Geometry check sheet. Reference: the model listing, model coordinates, mm. Face numbers are marked on the shaded views. A direction names the side the tool comes from. Coordinates: 2 decimals unless noted, no trailing zeros. Loops run counter-clockwise (first coordinate to the right, second up) from the corner with the lowest first, then second, coordinate; pieces in that order, holes last. Notation, with made-up numbers: (-30.5, 60.5) - (-2.5, 60.5) arc R19 cw to (-2.5, 92.5) - close; hole circle Ø11 at (70, 77.25). An arc over 180 degrees is marked (long way). One line per item, written item: value.
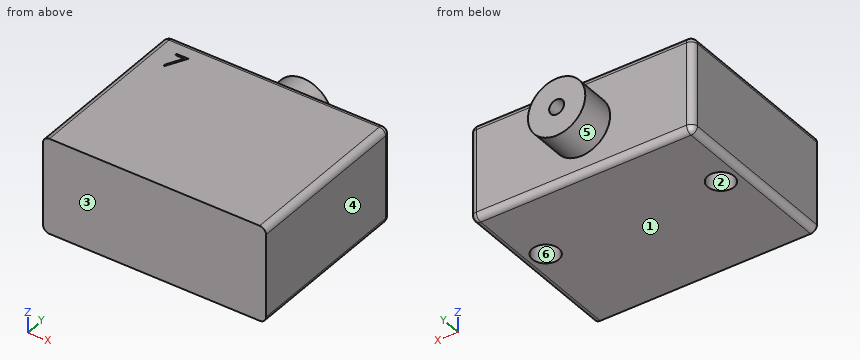
from build123d import *

# Parameters (mm, degrees)
CROQUIS1_W              = 70
CROQUIS1_H              = 30
SALIENTE_EXTRUIR1_DEPTH = 55
CROQUIS9_R              = 4.15
CORTAR_EXTRUIR6_DEPTH   = 27
REDONDEO1_R             = 2
CORTAR_EXTRUIR9_DEPTH   = 1
CROQUIS13_R             = 9
SALIENTE_EXTRUIR2_DEPTH = 11
CROQUIS14_R             = 2.35
CORTAR_EXTRUIR10_DEPTH  = 44


with BuildPart() as part:
    # Croquis1 → Saliente-Extruir1 (new body)
    with BuildSketch(Plane(origin=(0, 0, 0), x_dir=(1, 0, 0), z_dir=(0, 1, 0))):
        Rectangle(CROQUIS1_W, CROQUIS1_H)
    extrude(amount=SALIENTE_EXTRUIR1_DEPTH)

    # Croquis9 → Cortar-Extruir6 (cut)
    with BuildSketch(Plane(origin=(0, 0, -15), x_dir=(-1, 0, 0), z_dir=(0, 0, -1))):
        with Locations((-27.5, 32)):
            Circle(CROQUIS9_R)
        with Locations((27.5, 32)):
            Circle(CROQUIS9_R)
    extrude(amount=-CORTAR_EXTRUIR6_DEPTH, mode=Mode.SUBTRACT)

    # Redondeo1
    redondeo1_edges = [part.edges().sort_by_distance(p)[0] for p in [
        (-35, 55, 0),
        (0, 55, 15),
        (35, 55, 0),
        (0, 55, -15),
        (35, 27.5, 15),
        (-35, 27.5, 15),
        (-35, 27.5, -15),
        (35, 27.5, -15),
    ]]
    fillet(redondeo1_edges, radius=REDONDEO1_R)

    # Croquis12 → Cortar-Extruir9 (cut)
    with BuildSketch(Plane.XY.offset(15)):
        Polygon((-27.897004406, 49.221392525), (-24.204696713, 49.221392525), (-27.358542867, 43.067546371), (-27.823687098, 43.323555986), (-25.115754406, 48.606007909), (-27.897004406, 48.606007909), align=None)
    extrude(amount=-CORTAR_EXTRUIR9_DEPTH, mode=Mode.SUBTRACT)

    # Croquis13 → Saliente-Extruir2 (add)
    with BuildSketch(Plane(origin=(0, 55, 0), x_dir=(1, 0, 0), z_dir=(0, 1, 0))):
        with Locations(Location((0, 0, 0), (0, 0, 90))):
            Circle(CROQUIS13_R)
    extrude(amount=SALIENTE_EXTRUIR2_DEPTH)

    # Croquis14 → Cortar-Extruir10 (cut)
    with BuildSketch(Plane(origin=(0, 66, 0), x_dir=(1, 0, 0), z_dir=(0, 1, 0))):
        with Locations(Location((0, 0, 0), (0, 0, 270))):
            Circle(CROQUIS14_R)
    extrude(amount=-CORTAR_EXTRUIR10_DEPTH, mode=Mode.SUBTRACT)


solid = part.part
(1) Release check for a two-part mould opening along Y. For the marked faces 1, 2 and 3 record: pulls with the +Y half, pulls with the -Y half, needs draft (parallel to the pull), parting line crosses it, or undercut.
Reply:
face 1: needs draft
face 2: undercut
face 3: pulls with the -Y half
(2) Cross-section at A-A on y = 32. Record the cut outline in (x, z).
Reply:
outline: (-35, -13) arc R2 ccw to (-33, -15) - (-31.65, -15) - (-31.65, 12) - (-23.35, 12) - (-23.35, -15) - (23.35, -15) - (23.35, 12) - (31.65, 12) - (31.65, -15) - (33, -15) arc R2 ccw to (35, -13) - (35, 13) arc R2 ccw to (33, 15) - (-33, 15) arc R2 ccw to (-35, 13) - close; hole circle Ø4.7 at (0, 0)
(3) Go/stop test with flat-tipped pins: pin 1 Ø5 at (x, z) = (-18.5, 6) entering from +Y; pin 2 Ø7.5 at (x, y) = (27.5, 32) entering from -Z; pin 3 Ø1.1 at (x, z) = (-27, 14.5) entering from +Y. Record where each tip stops, or that it passes through.
Reply:
pin 1: y = 55
pin 2: z = 12
pin 3: y = 54.76
(4) Cross-section at D-D on z = 7.75. Record the cut outline in (x, y).
Reply:
outline: (-35, 0) - (35, 0) - (35, 53) arc R2 ccw to (33, 55) - (4.58, 55) - (4.58, 66) - (-4.58, 66) - (-4.58, 55) - (-33, 55) arc R2 ccw to (-35, 53) - close; hole circle Ø8.3 at (-27.5, 32); hole circle Ø8.3 at (27.5, 32)
(5) Material ranges on probe 1 along Y at (x, z) = (-27.5, -4.5); probe 2 along X at (y, z) = (47, 0); probe 3 along Y at (x, z) = (-23, 0.75), recorded low to high. Write a range as from..to.
Reply:
probe 1: 0..27.85, 36.15..55
probe 2: -35..-2.35, 2.35..35
probe 3: 0..55
(6) Cross-section at B-B on z = -4.25. Record the cut outline in (x, y).
Reply:
outline: (-35, 0) - (35, 0) - (35, 53) arc R2 ccw to (33, 55) - (7.93, 55) - (7.93, 66) - (-7.93, 66) - (-7.93, 55) - (-33, 55) arc R2 ccw to (-35, 53) - close; hole circle Ø8.3 at (-27.5, 32); hole circle Ø8.3 at (27.5, 32)
(7) Cross-section at C-C on x = 0. Record the cut outline in (y, z).
Reply:
outline: (0, -15) - (53, -15) arc R2 ccw to (55, -13) - (55, -9) - (66, -9) - (66, -2.35) - (22, -2.35) - (22, 2.35) - (66, 2.35) - (66, 9) - (55, 9) - (55, 13) arc R2 ccw to (53, 15) - (0, 15) - close
(8) Access from +Z, -Z, +X, -X, +Y, -Y to the whole of each face (thin tool, end or side, straight path). Record for the marked faces 4, 5 and 6.
Reply:
face 4: +Z, -Z, +X, +Y, -Y
face 5: +Y
face 6: -Z
